```python
from build123d import *

# Parameters (mm, degrees)
SKETCH1_W           = 80
SKETCH1_H           = 140
BOSS_EXTRUDE1_DEPTH = 3
SKETCH2_W           = 80
SKETCH2_H           = 140
SKETCH2_W_2         = 74
SKETCH2_H_2         = 134
BOSS_EXTRUDE2_DEPTH = 25
SKETCH3_R           = 1.6
BOSS_EXTRUDE3_DEPTH = 5
SKETCH4_W           = 80
SKETCH4_H           = 5
BOSS_EXTRUDE4_DEPTH = 2
CHAMFER1_SIZE       = 1
SKETCH5_R           = 4
CUT_EXTRUDE1_DEPTH  = 10
FILLET1_R           = 3


with BuildPart() as part:
    # Sketch1 → Boss-Extrude1 (new body)
    with BuildSketch(Plane(origin=(0, 0, 0), x_dir=(1, 0, 0), z_dir=(0, 1, 0))):
        Rectangle(SKETCH1_W, SKETCH1_H)
    extrude(amount=BOSS_EXTRUDE1_DEPTH)

    # Sketch2 → Boss-Extrude2 (add)
    with BuildSketch(Plane(origin=(0, 3, 0), x_dir=(1, 0, 0), z_dir=(0, 1, 0))):
        Rectangle(SKETCH2_W, SKETCH2_H)
        Rectangle(SKETCH2_W_2, SKETCH2_H_2, mode=Mode.SUBTRACT)
    extrude(amount=BOSS_EXTRUDE2_DEPTH)

    # Sketch3 → Boss-Extrude3 (add)
    with BuildSketch(Plane(origin=(0, 3, 0), x_dir=(1, 0, 0), z_dir=(0, 1, 0))):
        with Locations(Location((-23, 49, 0), (0, 0, 270))):
            Circle(SKETCH3_R)
        with Locations(Location((-23, 9, 0), (0, 0, 270))):
            Circle(SKETCH3_R)
        with Locations(Location((17, 9, 0), (0, 0, 90))):
            Circle(SKETCH3_R)
        with Locations(Location((17, 49, 0), (0, 0, 90))):
            Circle(SKETCH3_R)
    extrude(amount=BOSS_EXTRUDE3_DEPTH)

    # Sketch4 → Boss-Extrude4 (add)
    with BuildSketch(Plane.XZ):
        with Locations((0, -67.5)):
            Rectangle(SKETCH4_W, SKETCH4_H)
        with Locations((0, -55.3)):
            Rectangle(SKETCH4_W, SKETCH4_H)
        with Locations((0, -43.1)):
            Rectangle(SKETCH4_W, SKETCH4_H)
        with Locations((0, -30.9)):
            Rectangle(SKETCH4_W, SKETCH4_H)
        with Locations((0, -18.7)):
            Rectangle(SKETCH4_W, SKETCH4_H)
        with Locations((0, -6.5)):
            Rectangle(SKETCH4_W, SKETCH4_H)
        with Locations((0, 5.7)):
            Rectangle(SKETCH4_W, SKETCH4_H)
        with Locations((0, 17.9)):
            Rectangle(SKETCH4_W, SKETCH4_H)
        with Locations((0, 30.1)):
            Rectangle(SKETCH4_W, SKETCH4_H)
        with Locations((0, 42.3)):
            Rectangle(SKETCH4_W, SKETCH4_H)
        with Locations((0, 54.5)):
            Rectangle(SKETCH4_W, SKETCH4_H)
        with Locations((0, 66.7)):
            Rectangle(SKETCH4_W, SKETCH4_H)
    extrude(amount=BOSS_EXTRUDE4_DEPTH)

    # Chamfer1
    chamfer1_edges = [part.edges().sort_by_distance(p)[0] for p in [
        (0, -2, -16.2),
        (-40, -2, -6.5),
        (0, -2, -9),
        (40, -2, -6.5),
        (0, -2, -4),
        (-40, -2, 5.7),
        (0, -2, 3.2),
        (40, -2, 5.7),
        (0, -2, 8.2),
        (-40, -2, 17.9),
        (0, -2, 15.4),
        (40, -2, 17.9),
        (0, -2, 20.4),
        (-40, -2, 30.1),
        (0, -2, 27.6),
        (40, -2, 30.1),
        (0, -2, 32.6),
        (-40, -2, 42.3),
        (0, -2, 39.8),
        (40, -2, 42.3),
        (0, -2, 44.8),
        (-40, -2, 54.5),
        (0, -2, 52),
        (40, -2, 54.5),
        (0, -2, 57),
        (-40, -2, 66.7),
        (0, -2, 64.2),
        (40, -2, 66.7),
        (0, -2, 69.2),
        (-40, -2, -67.5),
        (0, -2, -70),
        (40, -2, -67.5),
        (0, -2, -65),
        (-40, -2, -55.3),
        (0, -2, -57.8),
        (40, -2, -55.3),
        (0, -2, -52.8),
        (-40, -2, -43.1),
        (0, -2, -45.6),
        (40, -2, -43.1),
        (0, -2, -40.6),
        (-40, -2, -30.9),
        (0, -2, -33.4),
        (40, -2, -30.9),
        (0, -2, -28.4),
        (-40, -2, -18.7),
        (0, -2, -21.2),
        (40, -2, -18.7),
    ]]
    chamfer(chamfer1_edges, length=CHAMFER1_SIZE)

    # Sketch5 → Cut-Extrude1 (cut)
    with BuildSketch(Plane(origin=(40, 0, 0), x_dir=(0, 0, -1), z_dir=(1, 0, 0))):
        with Locations((10, 8)):
            Circle(SKETCH5_R)
    extrude(amount=-CUT_EXTRUDE1_DEPTH, mode=Mode.SUBTRACT)

    # Fillet1
    # the kernel refuses this fillet: 3 mm, written as the material it takes off along each edge
    with BuildSketch(Plane(origin=(40, 35.5, 70), x_dir=(0, 0, -1), z_dir=(0, -1, 0)), Plane(origin=(-40, -7.5, 70), x_dir=(0, 0, -1), z_dir=(0, 1, 0))) as fillet1_piece_1:
        with BuildLine():
            CenterArc((FILLET1_R, -FILLET1_R), FILLET1_R, 90, 90)
            Line((0, -FILLET1_R), (0, 0))
            Line((0, 0), (FILLET1_R, 0))
        make_face()
    extrude(amount=43, mode=Mode.SUBTRACT)
    with BuildSketch(Plane(origin=(40, 35.5, -70), x_dir=(-1, 0, 0), z_dir=(0, -1, 0)), Plane(origin=(-40, -8.5, -70), x_dir=(1, 0, 0), z_dir=(0, 1, 0))) as fillet1_piece_2:
        with BuildLine():
            CenterArc((FILLET1_R, -FILLET1_R), FILLET1_R, 90, 90)
            Line((0, -FILLET1_R), (0, 0))
            Line((0, 0), (FILLET1_R, 0))
        make_face()
    extrude(amount=44, mode=Mode.SUBTRACT)


solid = part.part
```
The listing builds one solid part. Answer for the finished solid, in the listing's coordinates (mm). A direction names the side the tool comes from. Give positions to 0.01 mm unless a question says otherwise; leave off trailing zeros. Write each loop counter-clockwise with the first axis right and the second up, starting at its lowest first coordinate (ties: lowest second). Pieces come first, ordered by that corner, then holes. Notation, with made-up numbers: (-9, 35) - (36, 35) arc R9 cw to (36, 41) - close; hole circle Ø1 at (-30, 74). An arc over 180 degrees is marked (long way). Use one line per item in the form item = value. Start each with the question number.
1) A tool of negligible diameter and unlimited length cuts with its end or side. For faces 4 (the face through (-1, 0, 24)), 5 (the face through (-37, 15, 1)), 6 (the face through (-1, -2, 42)), from which of +Z, -Z, +X, -X, +Y, -Y can it reach the whole face along a straight path? Write none if from no direction.
2) Consider line 1 along X through (y, z) = (3.75, 44); line 2 along Z through (x, y) = (-16, 18.25); line 3 along Y through (x, z) = (39, -10). Determine where each line is inside the solid, lowest interval first. Write a range as from..to.
3) The mould has two halves that part along Y. Classify faces 1 (the face through (-1, 0, -37)), 2 (the face through (17, 8, -49)), 3 (the face through (38.5, 5.6, -6.8)): pulls with the +Y half, pulls with the -Y half, needs draft (parallel to the pull), parting line crosses it, or undercut.
4) Flat-ended cylindrical pins translate along their axes: pin 1 Ø2 at (x, z) = (7, -35.5) entering from -Y; pin 2 Ø0.5 at (x, y) = (1.5, -0.5) entering from +Z; pin 3 Ø1 at (x, z) = (7, 18) entering from +Y. Find the tip coordinate at first contact, or state that the pin passes through.
5) Find section A-A on y = 14. Determine the outline of the cut face in (x, z).
6) Find section B-B on z = -24.5. Determine the outline of the cut face in (x, y), plus the area to 3 significant figures.
Geometry results:
q1.face_4 = +X, -X, -Y
q1.face_5 = +Y
q1.face_6 = +Z, -Z, +X, -X, -Y
q2.line_1 = -40..-37, 37..40
q2.line_2 = -70..-67, 67..70
q2.line_3 = 0..4, 12..28
q3.face_1 = pulls with the -Y half
q3.face_2 = pulls with the +Y half
q3.face_3 = undercut
q4.pin_1 = 0
q4.pin_2 = 69.2
q4.pin_3 = 3
q5.outline = (-40, -67) arc R3 ccw to (-37, -70) - (37, -70) arc R3 ccw to (40, -67) - (40, 67) arc R3 ccw to (37, 70) - (-37, 70) arc R3 ccw to (-40, 67) - close; hole (-37, -67) - (37, -67) - (37, 67) - (-37, 67) - close
q6.outline = (-40, 0) - (40, 0) - (40, 28) - (37, 28) - (37, 3) - (-37, 3) - (-37, 28) - (-40, 28) - close
q6.area = 390 mm2
